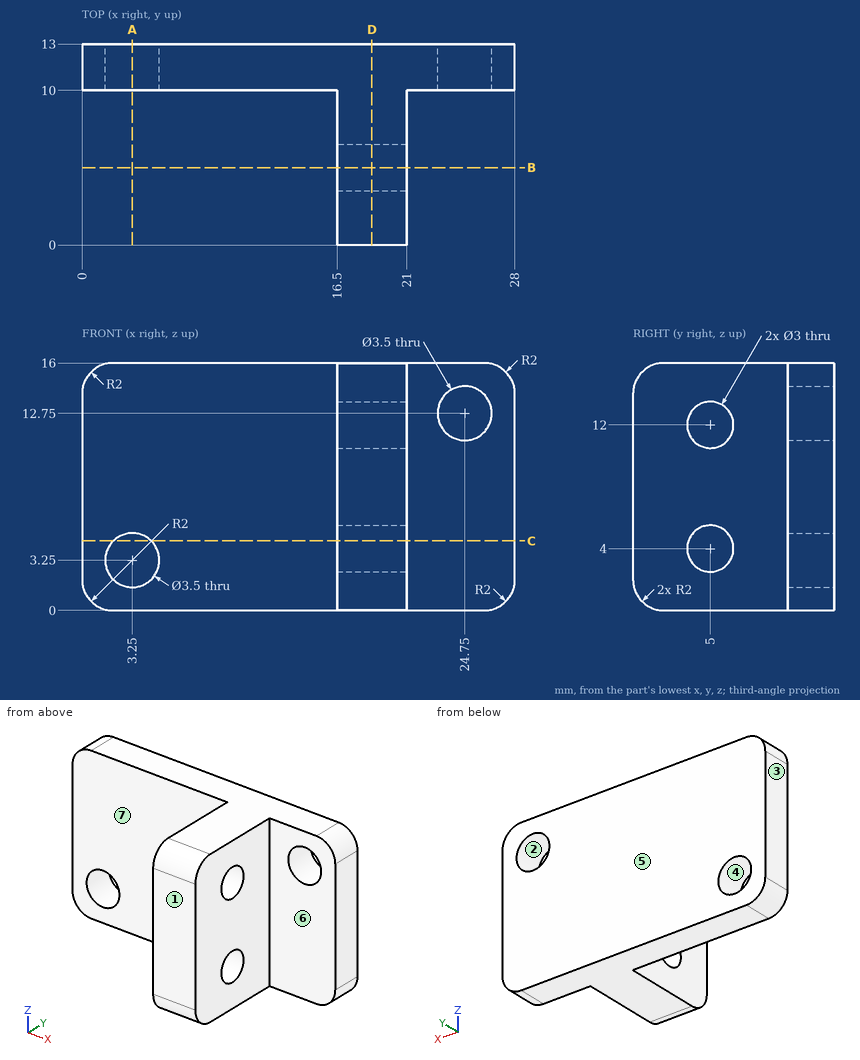
Design review of the part shown in the three views and the two pictorial views. Dimensions are in mm from the part's minimum x, y and z. A direction names the side the tool comes from. Give positions to 0.01 mm unless a question says otherwise; leave off trailing zeros. Write each loop counter-clockwise with the first axis right and the second up, starting at its lowest first coordinate (ties: lowest second). Pieces come first, ordered by that corner, then holes. Notation, with made-up numbers: (-36.75, -5.5) - (10.25, -5.5) arc R6 ccw to (10.25, -1.5) - close; hole circle Ø2 at (-19, 89.5). An arc over 180 degrees is marked (long way). Return JSON: item names as keys, results as strings. Group by question number.
(1) To check wall thickness, follow probe 1 along Z at (x, y) = (17.4, 5); probe 2 along Z at (x, y) = (17, 6); probe 3 along Z at (x, y) = (3.25, 12.1). State the ranges of each line that lie inside material, in increasing order.
(2) Mouldability with a two-part tool opening along X and no side actions: class the marked faces 1, 2, 3 and 4 as +X half, -X half, draft (parallel to the pull), parting line (faces both ways), or undercut.
(3) Insertion check: pin 1 (3.5 mm diameter, centred on y = 5, z = 4, fed in from -X); pin 2 (3 mm diameter, centred on x = 3.25, z = 3.25, fed in from -Y); pin 3 (8 mm diameter, centred on x = 8, z = 4.5, fed in from -Y); pin 4 (5 mm diameter, centred on y = 7, z = 9, fed in from +X). Each pin has a flat end and moves straight along its axis. Give the tip position at first contact, or say it passes through.
(4) We need section B-B, the plane y = 5. Give the boundary of the cut face in (x, z).
(5) We need section D-D, the plane x = 18.75. Give the boundary of the cut face in (y, z).
(6) Machinability: for the marked faces 5, 6 and 7, which of the approach directions +Z, -Z, +X, -X, +Y, -Y give a long, thin tool a straight path to every point of the face, cutting with its end or side? Answer none if there is none.
(7) We need section A-A, the plane x = 3.25. Give the boundary of the cut face in (y, z), then the cut area to 3 significant figures.
(8) We need section C-C, the plane z = 4.5. Give the boundary of the cut face in (x, y), then the cut area to 3 significant figures.
Reported:
{
 "1": {"probe 1": "z = 0 to 2.5, 5.5 to 10.5, 13.5 to 16", "probe 2": "z = 0 to 2.88, 5.12 to 10.88, 13.12 to 16", "probe 3": "z = 0 to 1.5, 5 to 16"},
 "2": {"face 1": "draft", "face 2": "undercut", "face 3": "-X half", "face 4": "undercut"},
 "3": {"pin 1": "stops at x = 16.5", "pin 2": "passes through", "pin 3": "stops at y = 10", "pin 4": "stops at x = 21"},
 "4": {"outline": "(16.5, 0) - (21, 0) - (21, 2.5) - (16.5, 2.5) - close; (16.5, 5.5) - (21, 5.5) - (21, 10.5) - (16.5, 10.5) - close; (16.5, 13.5) - (21, 13.5) - (21, 16) - (16.5, 16) - close"},
 "5": {"outline": "(0, 2) arc R2 ccw to (2, 0) - (13, 0) - (13, 16) - (2, 16) arc R2 ccw to (0, 14) - close; hole circle Ø3 at (5, 4); hole circle Ø3 at (5, 12)"},
 "6": {"face 5": "+Z, -Z, +X, -X, +Y", "face 6": "+Z, -Z, +X, -Y", "face 7": "+Z, -Z, -X, -Y"},
 "7": {"outline": "(10, 0) - (13, 0) - (13, 1.5) - (10, 1.5) - close; (10, 5) - (13, 5) - (13, 16) - (10, 16) - close", "area": "37.5 mm2"},
 "8": {"outline": "(0, 10) - (2.03, 10) - (2.03, 13) - (0, 13) - close; (4.47, 10) - (16.5, 10) - (16.5, 6.41) - (21, 6.41) - (21, 10) - (28, 10) - (28, 13) - (4.47, 13) - close; (16.5, 0) - (21, 0) - (21, 3.59) - (16.5, 3.59) - close", "area": "109 mm2"}
}
